Can you work these out from the model? Positions are in its coordinate system, mm. A direction names the side the tool comes from. Give positions to 0.01 mm unless a question says otherwise; leave off trailing zeros. Order: outer loops, then holes, each group sorted by start corner. A loop starts at its lowest first (then second) coordinate and runs counter-clockwise, first axis right, second up.
```python
from build123d import *

# Parameters (mm, degrees)
CROQUIS1_R              = 2.5
SALIENTE_EXTRUIR1_DEPTH = 26
CROQUIS2_R              = 1
CORTAR_EXTRUIR1_DEPTH   = 10
REDONDEO1_R             = 0.25


with BuildPart() as part:
    # Croquis1 → Saliente-Extruir1 (new body)
    with BuildSketch(Plane.XY):
        with Locations(Location((0, 0, 0), (0, 0, 180))):
            Circle(CROQUIS1_R)
    extrude(amount=SALIENTE_EXTRUIR1_DEPTH)

    # Croquis2 → Cortar-Extruir1 (cut)
    with BuildSketch(Plane.XY.offset(26)):
        Circle(CROQUIS2_R)
    extrude(amount=-CORTAR_EXTRUIR1_DEPTH, mode=Mode.SUBTRACT)

    # Redondeo1
    redondeo1_edges = [part.edges().sort_by_distance(p)[0] for p in [
        (2.5, 0, 26),
        (-1, 0, 26),
    ]]
    fillet(redondeo1_edges, radius=REDONDEO1_R)


solid = part.part
```
1) If I drill on line 1 (Y direction, x = 0, z = 20); line 2 (X direction, y = -0.15, z = 6.75); line 3 (X direction, y = -0.9, z = 22), over which ranges is the centre line in solid material (lowest first)?
2) Suppose I cut it at D-D (z = 11). Please give me the cut outline in (x, y), and give its area (3 significant figures).
3) Suppose I cut it at B-B (z = 19). Please give me the cut outline in (x, y), and give its area (3 significant figures).
4) Suppose I cut it at A-A (x = 0). Please give me the cut outline in (y, z), and give its area (3 significant figures).
5) Which directions (+Z, -Z, +X, -X, +Y, -Y) give clear straight access to the entire face, cutting with the end or side of a thin tool? Please do faces 1 (the face through (-1, 1, 26)), 2 (the face through (0, -1, 21)).
6) I'm going to push a flat-ended pin straight in: pin 1 Ø1.5 at (y, z) = (-2, 3.5) entering from -X. Where does the tip first touch, or does it pass through?
7) We'd pull the mould along Y, two halves only. Please class faces 3 (the face through (0, 0, 16)), 4 (the face through (2.5, -0.1, 12.7)), 5 (the face through (0, 0, 0)): +Y half, -Y half, draft (parallel to the pull), parting line (faces both ways), or undercut.
Results:
1. line 1: y = -2.5 to -1, 1 to 2.5
1. line 2: x = -2.5 to 2.5
1. line 3: x = -2.33 to -0.44, 0.44 to 2.33
2. outline: circle Ø5 at (0, 0)
2. area: 19.6 mm2
3. outline: circle Ø5 at (0, 0); hole circle Ø2 at (0, 0)
3. area: 16.5 mm2
4. outline: (-2.5, 0) - (2.5, 0) - (2.5, 25.75) arc R0.25 ccw to (2.25, 26) - (1.25, 26) arc R0.25 ccw to (1, 25.75) - (1, 16) - (-1, 16) - (-1, 25.75) arc R0.25 ccw to (-1.25, 26) - (-2.25, 26) arc R0.25 ccw to (-2.5, 25.75) - close
4. area: 110 mm2
5. face 1: +Z, +X, -X, +Y, -Y
5. face 2: +Z
6. pin 1: stops at x = -2.17
7. face 3: undercut
7. face 4: parting line
7. face 5: draft
